Model file for the job. Use its own axes, mm. Round coordinates to 2 decimals unless told otherwise and drop trailing zeros. Write each loop counter-clockwise with the first axis right and the second up, starting at its lowest first coordinate (ties: lowest second). Pieces come first, ordered by that corner, then holes.
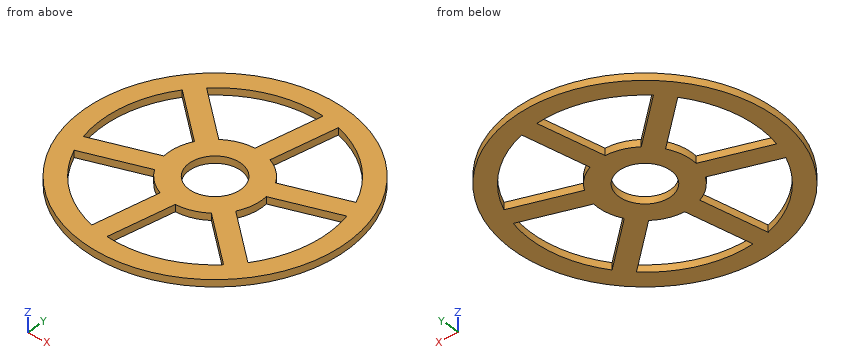
```python
from build123d import *

# Parameters (mm, degrees)
SKETCH1_R           = 88.9
SKETCH1_R_2         = 17.5
BOSS_EXTRUDE1_DEPTH = 4.7625


with BuildPart() as part:
    # Sketch1 → Boss-Extrude1 (new body)
    with BuildSketch(Plane.XY):
        with Locations(Location((0, 0, 0), (0, 0, 180))):
            Circle(SKETCH1_R)
        with Locations(Location((0, 0, 0), (0, 0, 180))):
            Circle(SKETCH1_R_2, mode=Mode.SUBTRACT)
        with BuildLine():
            Line((8.965287197, 75.670758061), (0, 31.75))
            ThreePointArc((0, 31.75), (-10.054998553, 30.115768363), (-19.074898098, 25.381307345))
            Line((-19.074898098, 25.381307345), (-52.628746733, 55.10585284))
            ThreePointArc((-52.628746733, 55.10585284), (-24.131996526, 72.277844072), (8.965287197, 75.670758061))
        make_face(mode=Mode.SUBTRACT)
        with BuildLine():
            Line((70.015442403, 30.071212565), (27.49630657, 15.875))
            ThreePointArc((27.49630657, 15.875), (21.053521181, 23.765768363), (12.443407893, 29.21))
            Line((12.443407893, 29.21), (21.40869509, 73.130758061))
            ThreePointArc((21.40869509, 73.130758061), (50.528450834, 57.037844072), (70.015442403, 30.071212565))
        make_face(mode=Mode.SUBTRACT)
        with BuildLine():
            Line((61.050155206, -45.599545495), (27.49630657, -15.875))
            ThreePointArc((27.49630657, -15.875), (31.108519733, -6.35), (31.518305991, 3.828692655))
            Line((31.518305991, 3.828692655), (74.037441824, 18.02490522))
            ThreePointArc((74.037441824, 18.02490522), (74.66044736, -15.24), (61.050155206, -45.599545495))
        make_face(mode=Mode.SUBTRACT)
        with BuildLine():
            Line((-8.965287197, -75.670758061), (0, -31.75))
            ThreePointArc((0, -31.75), (10.054998553, -30.115768363), (19.074898098, -25.381307345))
            Line((19.074898098, -25.381307345), (52.628746733, -55.10585284))
            ThreePointArc((52.628746733, -55.10585284), (24.131996526, -72.277844072), (-8.965287197, -75.670758061))
        make_face(mode=Mode.SUBTRACT)
        with BuildLine():
            Line((-70.015442403, -30.071212565), (-27.49630657, -15.875))
            ThreePointArc((-27.49630657, -15.875), (-21.053521181, -23.765768363), (-12.443407893, -29.21))
            Line((-12.443407893, -29.21), (-21.40869509, -73.130758061))
            ThreePointArc((-21.40869509, -73.130758061), (-50.528450834, -57.037844072), (-70.015442403, -30.071212565))
        make_face(mode=Mode.SUBTRACT)
        with BuildLine():
            Line((-61.050155206, 45.599545495), (-27.49630657, 15.875))
            ThreePointArc((-27.49630657, 15.875), (-31.108519733, 6.35), (-31.518305991, -3.828692655))
            Line((-31.518305991, -3.828692655), (-74.037441824, -18.02490522))
            ThreePointArc((-74.037441824, -18.02490522), (-74.66044736, 15.24), (-61.050155206, 45.599545495))
        make_face(mode=Mode.SUBTRACT)
    extrude(amount=BOSS_EXTRUDE1_DEPTH)


solid = part.part
```
1) Cut at A-A on y = 0. List the corners of the cut face in (x, z), and give its area (3 significant figures).
2) Cut at D-D on x = -55.5. List the corners of the cut face in (y, z).
3) Wall check: probe 1 along Y at (x, z) = (42.5, 1.05); probe 2 along X at (y, z) = (66, 1); probe 3 along Y at (x, z) = (57, 1.6). Give the ranges that are in metal, low to high.
4) Cut at C-C on x = 35. List the corners of the cut face in (y, z).
5) Cut at B-B on z = 1.55. List the corners of the cut face in (x, y) (3 decimals).
6) Flat gauge pins, fed straight in: pin 1 Ø1.5 at (y, z) = (10, 4) entering from -X; pin 2 Ø1.5 at (x, z) = (-58, 1) entering from +Y; pin 3 Ø1.5 at (y, z) = (-46, 4.5) entering from +X. Where does each tip first touch, or does it go through?
Result sheet:
1. outline: (-88.9, 0) - (-76.2, 0) - (-76.2, 4.76) - (-88.9, 4.76) - close; (-31.75, 0) - (-17.5, 0) - (-17.5, 4.76) - (-31.75, 4.76) - close; (17.5, 0) - (31.75, 0) - (31.75, 4.76) - (17.5, 4.76) - close; (76.2, 0) - (88.9, 0) - (88.9, 4.76) - (76.2, 4.76) - close
1. area: 257 mm2
2. outline: (-69.45, 0) - (-52.21, 0) - (-52.21, 4.76) - (-69.45, 4.76) - close; (-25.22, 0) - (-11.84, 0) - (-11.84, 4.76) - (-25.22, 4.76) - close; (40.68, 0) - (69.45, 0) - (69.45, 4.76) - (40.68, 4.76) - close
3. probe 1: y = -78.08 to -63.25, -46.13 to -29.17, 7.5 to 20.88, 63.25 to 78.08
3. probe 2: x = -59.56 to -38.08, 6.99 to 19.95, 38.08 to 59.56
3. probe 3: y = -68.22 to -42.01, 12.34 to 25.73, 50.57 to 68.22
4. outline: (-81.72, 0) - (-67.69, 0) - (-67.69, 4.76) - (-81.72, 4.76) - close; (-39.49, 0) - (-22.52, 0) - (-22.52, 4.76) - (-39.49, 4.76) - close; (4.99, 0) - (18.38, 0) - (18.38, 4.76) - (4.99, 4.76) - close; (67.69, 0) - (81.72, 0) - (81.72, 4.76) - (67.69, 4.76) - close
5. outline: circle Ø177.8 at (0, 0); hole (-74.037, -18.025) - (-31.518, -3.829) arc R31.75 cw to (-27.496, 15.875) - (-61.05, 45.6) arc R76.2 ccw to start; hole (-70.015, -30.071) arc R76.2 ccw to (-21.409, -73.131) - (-12.443, -29.21) arc R31.75 cw to (-27.496, -15.875) - close; hole (-52.629, 55.106) - (-19.075, 25.381) arc R31.75 cw to (0, 31.75) - (8.965, 75.671) arc R76.2 ccw to start; hole circle Ø35 at (0, 0); hole (-8.965, -75.671) arc R76.2 ccw to (52.629, -55.106) - (19.075, -25.381) arc R31.75 cw to (0, -31.75) - close; hole (12.443, 29.21) arc R31.75 cw to (27.496, 15.875) - (70.015, 30.071) arc R76.2 ccw to (21.409, 73.131) - close; hole (27.496, -15.875) - (61.05, -45.6) arc R76.2 ccw to (74.037, 18.025) - (31.518, 3.829) arc R31.75 cw to start
6. pin 1: stops at x = -88.42
6. pin 2: stops at y = 68.01
6. pin 3: stops at x = 76.52
